Source: CAD feature listing. Evaluate the final solid. Frame: model axes, mm. Face numbers are marked on the shaded views. A direction names the side the tool comes from. Round coordinates to 2 decimals unless told otherwise and drop trailing zeros. Loops run counter-clockwise (first coordinate to the right, second up) from the corner with the lowest first, then second, coordinate; pieces in that order, holes last. Notation, with made-up numbers: (36.25, 53) -> (51.25, 53) arc R7 ccw to (51.25, 60) -> close; hole circle Ø11 at (-22, 68). An arc over 180 degrees is marked (long way). Write item = value, one per line.
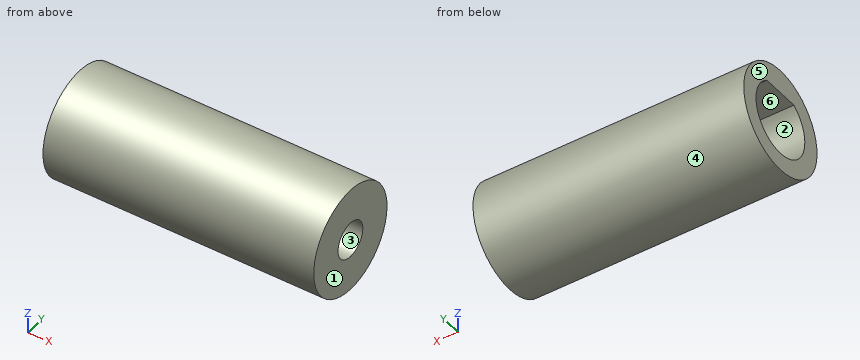
from build123d import *

# Parameters (mm, degrees)
SKETCH1_R           = 4.5
BOSS_EXTRUDE1_DEPTH = 14
SKETCH2_R           = 4.5
BOSS_EXTRUDE2_DEPTH = 2
SKETCH3_R           = 4.5
SKETCH3_R_2         = 1.525
BOSS_EXTRUDE3_DEPTH = 7


with BuildPart() as part:
    # Sketch1 → Boss-Extrude1 (new body)
    with BuildSketch(Plane.YZ):
        with Locations(Location((0, 0, 0), (0, 0, 270))):
            Circle(SKETCH1_R)
        with BuildLine():
            Line((-1.658312395, 2.5), (1.658312395, 2.5))
            ThreePointArc((1.658312395, 2.5), (0, -3), (-1.658312395, 2.5))
        make_face(mode=Mode.SUBTRACT)
    extrude(amount=BOSS_EXTRUDE1_DEPTH)

    # Sketch2 → Boss-Extrude2 (add)
    with BuildSketch(Plane.YZ.offset(14)):
        with Locations(Location((0, 0, 0), (0, 0, 270))):
            Circle(SKETCH2_R)
    extrude(amount=BOSS_EXTRUDE2_DEPTH)

    # Sketch3 → Boss-Extrude3 (add)
    with BuildSketch(Plane.YZ.offset(16)):
        with Locations(Location((0, 0, 0), (0, 0, 270))):
            Circle(SKETCH3_R)
        with Locations(Location((0, 0, 0), (0, 0, 270))):
            Circle(SKETCH3_R_2, mode=Mode.SUBTRACT)
    extrude(amount=BOSS_EXTRUDE3_DEPTH)


solid = part.part
1. Section query A-A (y = 0). Return the cut outline in (x, z) (3 decimals).
Evaluation:
outline = (0, -4.5) -> (23, -4.5) -> (23, -1.525) -> (16, -1.525) -> (16, 1.525) -> (23, 1.525) -> (23, 4.5) -> (0, 4.5) -> (0, 2.5) -> (14, 2.5) -> (14, -3) -> (0, -3) -> close
2. Section query D-D (x = 15). Return the cut outline in (y, z).
Evaluation:
outline = circle Ø9 at (0, 0)
3. Section query B-B (z = 0). Return the cut outline in (x, y) (3 decimals), then the cut area to 3 significant figures.
Evaluation:
outline = (0, -4.5) -> (23, -4.5) -> (23, -1.525) -> (16, -1.525) -> (16, 1.525) -> (23, 1.525) -> (23, 4.5) -> (0, 4.5) -> (0, 3) -> (14, 3) -> (14, -3) -> (0, -3) -> close
area = 102 mm²
4. Mould query, pull axis Y, two halves, no side actions, for the marked faces 3, 4, 5 and 6. Classes: released by +Y, released by -Y, zero draft, split by the parting line, or undercut.
Evaluation:
face_3 = undercut
face_4 = split by the parting line
face_5 = zero draft
face_6 = undercut
5. Section query C-C (x = 8.25). Return the cut outline in (y, z), then the cut area to 3 significant figures.
Evaluation:
outline = circle Ø9 at (0, 0); hole (-1.66, 2.5) arc R3 ccw (long way) to (1.66, 2.5) -> close
area = 36.5 mm²
6. Contact query for flat-ended pins moving along their axis: pin 1 Ø2.5 at (y, z) = (0, 0) entering from -X; pin 2 Ø2 at (x, z) = (15, -3.5) entering from -Y; pin 3 Ø1.5 at (y, z) = (-0.5, 0) entering from +X. Output: stop coordinate, or through.
Evaluation:
pin_1 = 14
pin_2 = -3.74
pin_3 = 16
7. Set-up query: the marked faces 1 and 2. Return all of +Z, -Z, +X, -X, +Y, -Y with unobstructed straight access to the full face (end or side cutting, diameter ignored); none if empty.
Evaluation:
face_1 = +Z, -Z, +X, +Y, -Y
face_2 = -X
8. Line query: probe 1 along Y at (x, z) = (4.5, 0); probe 2 along Y at (x, z) = (19, 0) (3 decimals); probe 3 along Z at (x, y) = (13.25, 1). Output: solid intervals per line, ascending. Write a range as from..to.
Evaluation:
probe_1 = -4.5..-3, 3..4.5
probe_2 = -4.5..-1.525, 1.525..4.5
probe_3 = -4.39..-2.83, 2.5..4.39
